```python
from build123d import *

# Parameters (mm, degrees)
F0_W           = 101.6
F0_H           = 50.8
F1_DEPTH       = 12.7
F2_SIZE        = 1.5875
F4_D           = 3.175
F4_CBORE_D     = 6.35
F4_CBORE_DEPTH = 3.175
F6_DEPTH       = 101.601
F7_W           = 3.175
F7_H           = 24.839708
F8_DEPTH       = 101.6


with BuildPart() as f1:
    # F0 (on Front) → F1 (new body)
    with BuildSketch(Plane.XZ):
        with Locations((50.8, 25.4)):
            Rectangle(F0_W, F0_H)
    extrude(amount=F1_DEPTH)

    # F2
    f2_edges = [f1.edges().sort_by_distance(p)[0] for p in [
        (50.8, -12.7, 50.8),
        (50.8, -12.7, 0),
    ]]
    chamfer(f2_edges, length=F2_SIZE)

    # F4 (through all)
    with Locations(Plane.XZ.offset(12.7)):
        with Locations((6.35, 6.35), (6.35, 44.45), (95.25, 44.45), (95.25, 6.35)):
            CounterBoreHole(F4_D / 2, F4_CBORE_D / 2, F4_CBORE_DEPTH)

    # F5 (on face) → F6 (cut, through all)
    with BuildSketch(Plane(origin=(0, 0, 0), x_dir=(0, -1, 0), z_dir=(-1, 0, 0))):
        Polygon((12.7, 17.1958), (12.7, 33.6042), (8.2042, 38.1), (8.2042, 12.7), align=None)
    extrude(amount=-F6_DEPTH, mode=Mode.SUBTRACT)

    # F7 (on face) → F8 (cut, through all)
    with BuildSketch(Plane(origin=(0, 0, 0), x_dir=(0, -1, 0), z_dir=(-1, 0, 0))):
        with Locations((1.5875, 25.119854)):
            Rectangle(F7_W, F7_H)
    extrude(amount=-F8_DEPTH, mode=Mode.SUBTRACT)


solid = f1.part
```
Verification items for the finished model (mm, model axes). A direction names the side the tool comes from. Round coordinates to 2 decimals unless told otherwise and drop trailing zeros. Loops run counter-clockwise (first coordinate to the right, second up) from the corner with the lowest first, then second, coordinate; pieces in that order, holes last. Notation, with made-up numbers: (-19, -16.5) -> (30, -16.5) arc R18 cw to (30, 9.5) -> close; hole circle Ø4 at (16.25, -21.5). An arc over 180 degrees is marked (long way). Answer as a JSON object with one key per item and string values.
Q1. Section check D-D (z = 36). Record the boundary of the cut face in (x, y) (3 decimals), then the cut area to 3 significant figures.
Data:
{"outline": "(0, -12.7) -> (101.6, -12.7) -> (101.6, -10.304) -> (0, -10.304) -> close; (0, -8.204) -> (101.6, -8.204) -> (101.6, -3.175) -> (0, -3.175) -> close", "area": "754 mm2"}
Q2. Go/stop test with flat-tipped pins: P1, Ø12.5, axis at x = 48, z = 23.5, coming from the +Y side (3 decimals); P2, Ø3, axis at x = 7.5, z = 45, coming from the -Y side (3 decimals). Record where each tip stops, or that it passes through.
Data:
{"P1": "stops at y = -3.175", "P2": "stops at y = -9.525"}
Q3. Draft check along Y on faces 4 (the flat face through (50.089, -10.421, 14.916)), 5 (the flat face through (50, -12.7, 42)), 6 (the flat face through (101.6, -6, 25)). Enter one of: pulls with the +Y half, pulls with the -Y half, needs draft (parallel to the pull), parting line crosses it, or undercut.
Data:
{"face 4": "undercut", "face 5": "pulls with the -Y half", "face 6": "needs draft"}
Q4. Section check C-C (x = 43.5). Record the boundary of the cut face in (y, z) (1 decimal), then the cut area to 3 significant figures.
Data:
{"outline": "(-12.7, 1.6) -> (-11.1, 0) -> (0, 0) -> (0, 12.7) -> (-3.2, 12.7) -> (-3.2, 37.5) -> (0, 37.5) -> (0, 50.8) -> (-11.1, 50.8) -> (-12.7, 49.2) -> (-12.7, 33.6) -> (-8.2, 38.1) -> (-8.2, 12.7) -> (-12.7, 17.2) -> close", "area": "470 mm2"}
Q5. Access from +Z, -Z, +X, -X, +Y, -Y to the whole of each face (thin tool, end or side, straight path). Record for faces 1 (the cylindrical face through (98.28, -11.13, 7.3)), 2 (the flat face through (50, -3.175, 25)), 3 (the flat face through (50, -5, 50.8)).
Data:
{"face 1": "-Y", "face 2": "+X, -X, +Y", "face 3": "+Z, +X, -X, +Y, -Y"}
Q6. Section check A-A (x = 6.35). State how many separate pieces and enclosed holes the cut face has, then the cut area to 3 significant figures.
Data:
{"separate pieces": "3", "enclosed holes": "0", "area": "369 mm2"}
Q7. Section check B-B (z = 6.35). Record the boundary of the cut face in (x, y) (1 decimal), then the cut area to 3 significant figures.
Data:
{"outline": "(0, -12.7) -> (3.2, -12.7) -> (3.2, -9.5) -> (4.8, -9.5) -> (4.8, 0) -> (0, 0) -> close; (7.9, -9.5) -> (9.5, -9.5) -> (9.5, -12.7) -> (92.1, -12.7) -> (92.1, -9.5) -> (93.7, -9.5) -> (93.7, 0) -> (7.9, 0) -> close; (96.8, -9.5) -> (98.4, -9.5) -> (98.4, -12.7) -> (101.6, -12.7) -> (101.6, 0) -> (96.8, 0) -> close", "area": "1,190 mm2"}
Q8. Scan lines: line 1 (Z direction, x = 6.35, y = -4.25); line 2 (Z direction, x = 6.35, y = -3); line 3 (Z direction, x = 6.35, y = -11.7) (1 decimal). Record each from-to range of solid material in increasing order. Write a range as from..to.
Data:
{"line 1": "z = 0..4.76, 7.94..42.86, 46.04..50.8", "line 2": "z = 0..4.76, 7.94..12.7, 37.54..42.86, 46.04..50.8", "line 3": "z = 0.6..3.2, 9.5..16.2, 34.6..41.3, 47.6..50.2"}
